For this review, use the dimensioned drawing (mm, ordinates from the lowest corner) and the shaded views. Round coordinates to 2 decimals unless told otherwise and drop trailing zeros. Write each loop counter-clockwise with the first axis right and the second up, starting at its lowest first coordinate (ties: lowest second). Pieces come first, ordered by that corner, then holes.
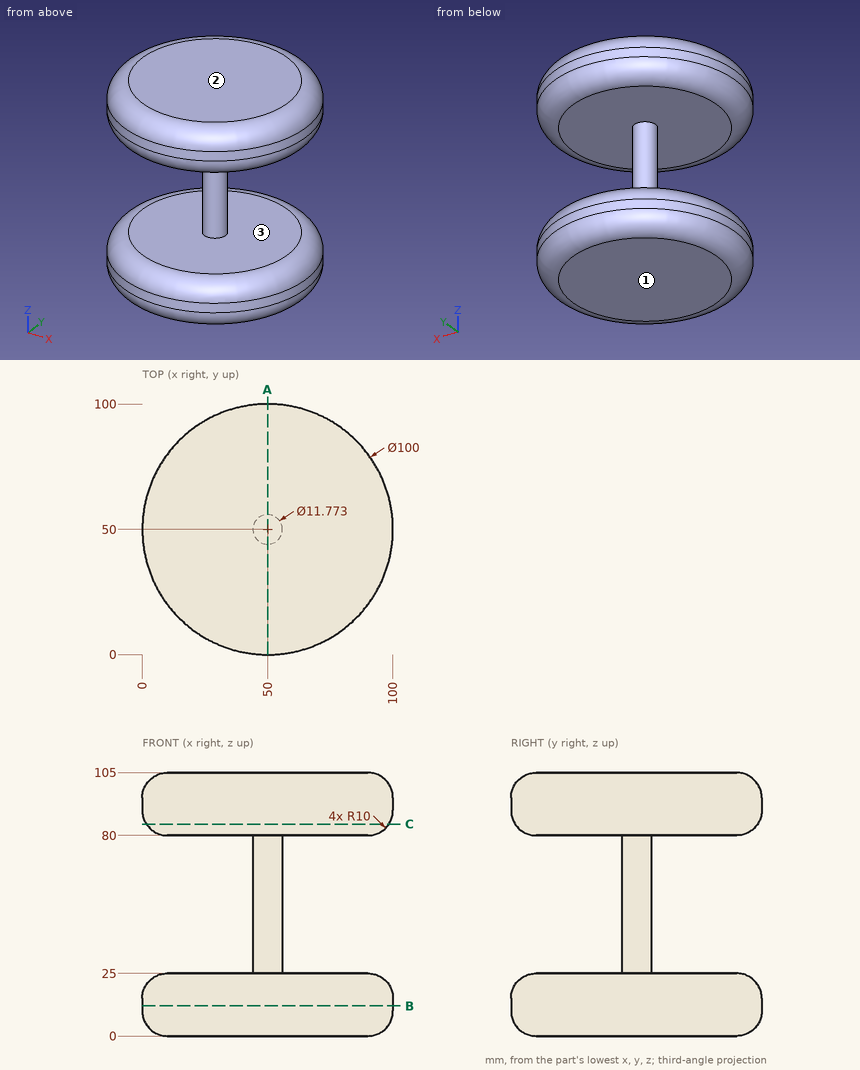
(1) For pin 1 Ø5 at (x, z) = (11, 76) entering from +Y; pin 2 Ø2 at (x, z) = (64, 11.5) entering from +Y; pin 3 Ø3 at (y, z) = (71, 20) entering from +X, all flat-tipped, find the tip position at first contact; note any pin that passes through.
Geometry check:
pin 1: passes through
pin 2: stops at y = 98.28
pin 3: stops at x = 94.97
(2) Mouldability with a two-part tool opening along Z and no side actions: class the marked faces 1, 2 and 3 as pulls with the +Z half, pulls with the -Z half, needs draft (parallel to the pull), parting line crosses it, or undercut.
Geometry check:
face 1: pulls with the -Z half
face 2: pulls with the +Z half
face 3: undercut
(3) For line 1 along Z through (x, y) = (73, 56); line 2 along Z through (x, y) = (7, 28.5); line 3 along Y through (x, z) = (74, 16), list the stretches that pass through material, from the lowest coordinate up.
Geometry check:
line 1: z = 0 to 25, 80 to 105
line 2: z = 4.1 to 20.9, 84.1 to 100.9
line 3: y = 6.19 to 93.81
(4) We need section C-C, the plane z = 84.5. Give the boundary of the cut face in (x, y), and give its area (3 significant figures).
Geometry check:
outline: circle Ø96.7 at (50, 50)
area: 7,340 mm2
(5) We need section B-B, the plane z = 12. Give the boundary of the cut face in (x, y), and give its area (3 significant figures).
Geometry check:
outline: circle Ø100 at (50, 50)
area: 7,850 mm2
(6) We need section A-A, the plane x = 50. Give the boundary of the cut face in (y, z).
Geometry check:
outline: (0, 10) arc R10 ccw to (10, 0) - (90, 0) arc R10 ccw to (100, 10) - (100, 15) arc R10 ccw to (90, 25) - (55.89, 25) - (55.89, 80) - (90, 80) arc R10 ccw to (100, 90) - (100, 95) arc R10 ccw to (90, 105) - (10, 105) arc R10 ccw to (0, 95) - (0, 90) arc R10 ccw to (10, 80) - (44.11, 80) - (44.11, 25) - (10, 25) arc R10 ccw to (0, 15) - close
